from build123d import *

# Parameters (mm, degrees)
SCHIZZO1_W                      = 300
SCHIZZO1_H                      = 20
ESTRUSIONE_ESTRUSIONE1_DEPTH    = 10
FORO_FILETTATO_M6_1_D           = 5
FORO_FILETTATO_M6_1_DEPTH       = 11
FORO_FILETTATO_M6_1_CSINK_D     = 7
FORO_FILETTATO_M6_1_CSINK_ANGLE = 90
FORO_FILETTATO_M6_1_TIP         = 1.502151548
RACCORDO1_R                     = 5


with BuildPart() as part:
    # Schizzo1 → Estrusione-Estrusione1 (new body)
    with BuildSketch(Plane(origin=(0, 0, 0), x_dir=(1, 0, 0), z_dir=(0, 1, 0))):
        Rectangle(SCHIZZO1_W, SCHIZZO1_H)
    extrude(amount=ESTRUSIONE_ESTRUSIONE1_DEPTH)

    # Foro filettato M6-1
    with Locations(Plane(origin=(0, 10, 0), x_dir=(-1, 0, 0), z_dir=(0, 1, 0))):
        with Locations((140, 0), (-140, 0)):
            CounterSinkHole(FORO_FILETTATO_M6_1_D / 2, FORO_FILETTATO_M6_1_CSINK_D / 2, depth=FORO_FILETTATO_M6_1_DEPTH, counter_sink_angle=FORO_FILETTATO_M6_1_CSINK_ANGLE)
            with Locations((0, 0, -(FORO_FILETTATO_M6_1_DEPTH + FORO_FILETTATO_M6_1_TIP / 2))):  # 118° drill point
                Cone(0, FORO_FILETTATO_M6_1_D / 2, FORO_FILETTATO_M6_1_TIP, mode=Mode.SUBTRACT)

    # Raccordo1
    raccordo1_edges = [part.edges().sort_by_distance(p)[0] for p in [
        (-150, 5, -10),
        (150, 5, -10),
        (150, 5, 10),
        (-150, 5, 10),
    ]]
    fillet(raccordo1_edges, radius=RACCORDO1_R)


solid = part.part
Read the model definition and answer for the solid it produces. Units are mm, in the model's axes. Give positions to 0.01 mm unless a question says otherwise; leave off trailing zeros. Loops run counter-clockwise (first coordinate to the right, second up) from the corner with the lowest first, then second, coordinate; pieces in that order, holes last. Notation, with made-up numbers: (27, -39) - (38, -39) arc R23 ccw to (38, -29) - close; hole circle Ø8 at (84.5, 28.25). An arc over 180 degrees is marked (long way). Answer as CSV lines item,"result". Start each with the question number.
1) Each of these flat-tipped pins is pushed along its axis until it touches: pin 1 Ø4 at (y, z) = (7.5, -8) entering from -X; pin 2 Ø6 at (x, z) = (140, 0) entering from +Y. Where does it stop, or does it pass through?
2) Determine the mould class of faces 1 (the face through (-137.615, 4.437, 0.751)), 2 (the face through (149, 5, -8)), 3 (the face through (-150, 5, 0)) for opening direction X: released by +X, released by -X, zero draft, split by the parting line, or undercut.
3) Find section A-A (z = 0). Write down the section's boundary in (x, y).
4) Find section B-B (x = 140). Write down the section's boundary in (y, z).
5) Straight lines are drawn through the part: L1, parallel to X at y = 6, z = 0; L2, parallel to Z at x = -140, y = 7.25; L3, parallel to X at y = 5.75, z = 5.5. For each, find the intervals that lie inside material, in ascending order. Write a range as from..to.
Findings below:
1,pin 1,"x = -149.9"
1,pin 2,"y = 9.5"
2,face 1,"undercut"
2,face 2,"released by +X"
2,face 3,"released by -X"
3,outline,"(-150, 0) - (-142.5, 0) - (-142.5, 9) - (-143.5, 10) - (-150, 10) - close; (-137.5, 0) - (137.5, 0) - (137.5, 9) - (136.5, 10) - (-136.5, 10) - (-137.5, 9) - close; (142.5, 0) - (150, 0) - (150, 10) - (143.5, 10) - (142.5, 9) - close"
4,outline,"(0, -10) - (10, -10) - (10, -3.5) - (9, -2.5) - (0, -2.5) - close; (0, 2.5) - (9, 2.5) - (10, 3.5) - (10, 10) - (0, 10) - close"
5,L1,"-150..-142.5, -137.5..137.5, 142.5..150"
5,L2,"-10..-2.5, 2.5..10"
5,L3,"-149.97..149.97"
